Geometry check sheet. Reference: the model listing, model coordinates, mm. Give positions to 0.01 mm unless a question says otherwise; leave off trailing zeros. Use a Markdown table: item, result. Add a question column.
1. Depth check by flat-ended pin: P1, Ø10, axis at x = -39, y = 3, coming from the -Z side; P2, Ø1, axis at y = 22.5, z = 1, coming from the +X side; P3, Ø1, axis at x = -17, z = 1.5, coming from the +Y side; P4, Ø1, axis at y = 20.5, z = 1, coming from the -X side. Enter the tip coordinate at first touch or a pass-through.
2. Material ranges on L1, parallel to X at y = 2.54, z = 0.25; L2, parallel to X at y = 22, z = 0.65; L3, parallel to X at y = 38.5, z = 0.75, recorded low to high.
3. Cross-section at A-A on y = 21. Count the separate pieces of the cut face and the enclosed holes in it, and give its area (3 significant figures).
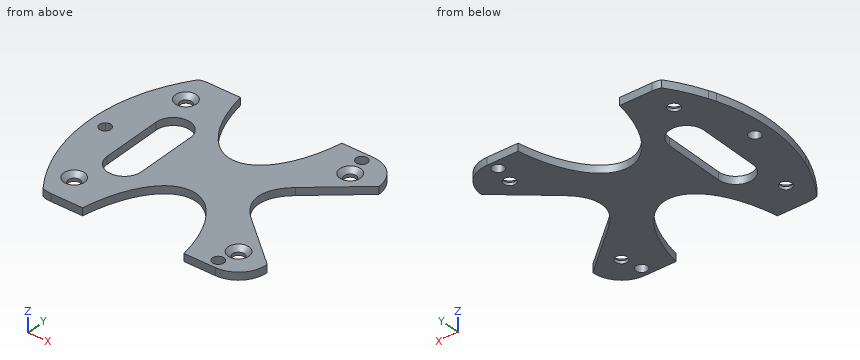
from build123d import *
from build123d.topology import SkipClean

# Parameters (mm, degrees)
BOSS_EXTRU_1_DEPTH                         = 2
FRAISAGE_POUR_VIS_T_TE_FRAIS_E_BOM_2_COUNT = 2
FRAISAGE_POUR_VIS_T_TE_FRAIS_E_BOM_2_PITCH = 36.576
FRAISAGE_POUR_VIS_T_TE_FRAIS_E_BOM_3_COUNT = 2
FRAISAGE_POUR_VIS_T_TE_FRAIS_E_BOM_3_PITCH = 56.589011089
FRAISAGE_POUR_VIS_T_TE_FRAIS_E_BOM_4_COUNT = 2
FRAISAGE_POUR_VIS_T_TE_FRAIS_E_BOM_4_PITCH = 43.18
ESQUISSE15_R                               = 1.5
ENL_V_MAT_EXTRU_5_DEPTH                    = 2
BOSS_EXTRU_3_DEPTH                         = 2
ENL_V_MAT_EXTRU_4_DEPTH                    = 2


with BuildPart() as part:
    # Esquisse1 → Boss.-Extru.1 (new body)
    with BuildSketch(Plane.XY):
        with BuildLine():
            Line((5, 2.54), (5, 39.116))
            ThreePointArc((5, 39.116), (2.79158513, 44.44758513), (-2.54, 46.656))
            Line((-2.54, 46.656), (-45.974, 46.656))
            ThreePointArc((-45.974, 46.656), (-51.125980008, 44.521980008), (-53.26, 39.37))
            Line((-53.26, 39.37), (-53.26, 2.54))
            ThreePointArc((-53.26, 2.54), (-51.05158513, -2.79158513), (-45.72, -5))
            Line((-45.72, -5), (-2.54, -5))
            ThreePointArc((-2.54, -5), (2.79158513, -2.79158513), (5, 2.54))
        make_face()
    extrude(amount=BOSS_EXTRU_1_DEPTH)

    # Esquisse16 → Fraisage pour vis à tête fraisée bombée M2.51 (revolve, cut)
    with BuildSketch(Plane(origin=(-2.54, 2.54, 2), x_dir=(0, -1, 0), z_dir=(1, 0, 0))):
        Polygon((0, 0), (0, 2), (1.55, 2), (1.55, 1.2), (2.75, 0), align=None)
    fraisage_pour_vis_t_te_frais_e_bomb_e = revolve(axis=Axis((-2.54, 2.54, 8.35), (0, 0, -1)), mode=Mode.SUBTRACT)

    # Fraisage pour vis _ t_te frais_e bom 2: Fraisage pour vis à tête fraisée bombée M2.51 ×2
    with Locations(*[(0, i * FRAISAGE_POUR_VIS_T_TE_FRAIS_E_BOM_2_PITCH, 0) for i in range(1, FRAISAGE_POUR_VIS_T_TE_FRAIS_E_BOM_2_COUNT)]):
        add(fraisage_pour_vis_t_te_frais_e_bomb_e, mode=Mode.SUBTRACT)

    # Fraisage pour vis _ t_te frais_e bom 3: Fraisage pour vis à tête fraisée bombée M2.51 ×2
    with Locations(*[Vector(-0.7630456721058034, 0.6463445693131512, 0) * (i * FRAISAGE_POUR_VIS_T_TE_FRAIS_E_BOM_3_PITCH) for i in range(1, FRAISAGE_POUR_VIS_T_TE_FRAIS_E_BOM_3_COUNT)]):
        add(fraisage_pour_vis_t_te_frais_e_bomb_e, mode=Mode.SUBTRACT)

    # Fraisage pour vis _ t_te frais_e bom 4: Fraisage pour vis à tête fraisée bombée M2.51 ×2
    with Locations(*[(-i * FRAISAGE_POUR_VIS_T_TE_FRAIS_E_BOM_4_PITCH, 0, 0) for i in range(1, FRAISAGE_POUR_VIS_T_TE_FRAIS_E_BOM_4_COUNT)]):
        add(fraisage_pour_vis_t_te_frais_e_bomb_e, mode=Mode.SUBTRACT)

    # Esquisse15 → Enlèv. mat.-Extru.5 (cut)
    with BuildSketch(Plane.XY):
        with Locations((-3.658386169, 44.310446006)):
            Circle(ESQUISSE15_R)
        with Locations((-52.330547462, 20.925047052)):
            Circle(ESQUISSE15_R)
        with Locations((-3.763486561, -2.551663742)):
            Circle(ESQUISSE15_R)
    extrude(amount=ENL_V_MAT_EXTRU_5_DEPTH, mode=Mode.SUBTRACT)

    # Esquisse14 → Boss.-Extru.3 (add)
    with BuildSketch(Plane.XY):
        with BuildLine():
            Line((-53.26, 22.10238217), (-53.26, 37.165169918))
            ThreePointArc((-53.26, 37.165169918), (-53.588975101, 36.32688135), (-53.900520078, 35.481960013))
            ThreePointArc((-53.900520078, 35.481960013), (-56.432053148, 20.831365998), (-53.880132923, 6.184309371))
            ThreePointArc((-53.880132923, 6.184309371), (-53.578203562, 5.368091645), (-53.26, 4.558079787))
            Line((-53.26, 4.558079787), (-53.26, 19.747711934))
            ThreePointArc((-53.26, 19.747711934), (-53.830547462, 20.925047052), (-53.26, 22.10238217))
        make_face()
    extrude(amount=BOSS_EXTRU_3_DEPTH)

    # Esquisse14<5> → Enlèv. mat.-Extru.4 (cut)
    with SkipClean():  # the faces are left unmerged after this step: merging them gives an invalid solid
        with BuildSketch(Plane.XY):
            with BuildLine():
                ThreePointArc((-53.26, 37.165169918), (-51.011337475, 41.886482774), (-48.212169147, 46.303714363))
                ThreePointArc((-48.212169147, 46.303714363), (-51.69919041, 43.876438812), (-53.239451379, 39.916820138))
                Line((-53.239451379, 39.916820138), (-53.900520078, 35.481960013))
                ThreePointArc((-53.900520078, 35.481960013), (-53.588975101, 36.32688135), (-53.26, 37.165169918))
            make_face()
            with BuildLine():
                add(Edge.make_bspline(
                    [(-37.449667929, 46.656), (-24.13, -31.756310028), (-10.810332071, 46.656)],
                    knots=[5.033406034, 5.033406034, 5.033406034, 7.53296458, 7.53296458, 7.53296458], degree=2, weights=[1, 0.315531822, 1]))
                Line((-10.810332071, 46.656), (-37.449667929, 46.656))
            make_face()
            with BuildLine():
                Line((-37.449667929, -5), (-10.810332071, -5))
                add(Edge.make_bspline(
                    [(-10.810332071, -5), (-24.13, 73.412310028), (-37.449667929, -5)],
                    knots=[5.033406034, 5.033406034, 5.033406034, 7.53296458, 7.53296458, 7.53296458], degree=2, weights=[1, 0.315531822, 1]))
            make_face()
            with BuildLine():
                ThreePointArc((-53.210302169, 1.675723757), (-51.610678888, -2.166538244), (-48.2162601, -4.574793427))
                ThreePointArc((-48.2162601, -4.574793427), (-51.013027883, -0.160172479), (-53.26, 4.558079787))
                ThreePointArc((-53.26, 4.558079787), (-53.578203562, 5.368091645), (-53.880132923, 6.184309371))
                Line((-53.880132923, 6.184309371), (-53.210302169, 1.675723757))
            make_face()
            with BuildLine():
                Line((-36.280356092, 12.815116729), (-36.280356092, 28.840883271))
                ThreePointArc((-36.280356092, 28.840883271), (-40.789570049, 33.350097228), (-45.298784007, 28.840883271))
                Line((-45.298784007, 28.840883271), (-45.298784007, 12.815116729))
                ThreePointArc((-45.298784007, 12.815116729), (-40.789570049, 8.305902772), (-36.280356092, 12.815116729))
            make_face()
            with BuildLine():
                Line((5, 39.116), (-8.045410448, 28.091494556))
                add(Edge.make_bspline(
                    [(-8.045410448, 28.091494556), (-16.636453297, 20.831316808), (-8.047692631, 13.570434437)],
                    knots=[5.739468015, 5.739468015, 5.739468015, 6.826742025, 6.826742025, 6.826742025], degree=2, weights=[1, 0.855833098, 1]))
                Line((-8.047692631, 13.570434437), (5, 2.54))
                Line((5, 2.54), (5, 39.116))
            make_face()
        extrude(amount=ENL_V_MAT_EXTRU_4_DEPTH, mode=Mode.SUBTRACT)


solid = part.part
Values found:
| question | item | result |
|---|---|---|
| 1 | P1 | stops at z = 0 |
| 1 | P2 | stops at x = -11.68 |
| 1 | P3 | stops at y = 32.26 |
| 1 | P4 | stops at x = -56.43 |
| 2 | L1 | x = -52.38 to -47.27, -44.17 to -35.46, -12.8 to -4.09, -0.99 to 5 |
| 2 | L2 | x = -56.42 to -53.38, -51.28 to -45.3, -36.28 to -11.91 |
| 2 | L3 | x = -52.69 to -47.14, -44.3 to -35.23, -13.03 to -3.96, -1.12 to 4.27 |
| 3 | separate pieces | 3 |
| 3 | enclosed holes | 0 |
| 3 | area | 64.8 mm2 |
